Model file for the job. Use its own axes, mm. Give positions to 0.01 mm unless a question says otherwise; leave off trailing zeros. Loops run counter-clockwise (first coordinate to the right, second up) from the corner with the lowest first, then second, coordinate; pieces in that order, holes last. Notation, with made-up numbers: (-29, 0) -> (-20, 0) arc R20 cw to (-20, 23) -> close; hole circle Ø11 at (33.25, -10.5). An arc over 180 degrees is marked (long way). Use CSV: the item, a comma, the result in double quotes. Start each with the question number.
(1) Flat gauge pins, fed straight in: pin 1 (3.5 mm diameter, centred on x = -2.88, y = -6.38, fed in from -Z); pin 2 (8 mm diameter, centred on y = -72.5, z = 27.5, fed in from -X); pin 3 (13.5 mm diameter, centred on x = 21.5, y = -71, fed in from +Z). Where does each tip first touch, or does it go through?
(2) Cut at B-B on x = 21. Write the cut outline in (y, z), then the cut area to 3 significant figures.
(3) Drill centre lines: probe 1 along Z at (x, y) = (-14, -10); probe 2 along Y at (x, z) = (90.5, 5); probe 3 along Y at (x, z) = (67, -17). Where is each one in solid material? Low to high.
(4) Cut at A-A on x = -17. Write the cut outline in (y, z), then the cut area to 3 significant figures.
from build123d import *

# Parameters (mm, degrees)
SKETCH2_R           = 10
SKETCH2_R_2         = 1.275
BOSS_EXTRUDE1_DEPTH = 3
SKETCH3_R           = 1.275
BOSS_EXTRUDE2_DEPTH = 5
BOSS_EXTRUDE3_DEPTH = 5


with BuildPart() as part:
    # Sketch2 → Boss-Extrude1 (new body)
    with BuildSketch(Plane.XY):
        Circle(SKETCH2_R)
        with Locations((2.883236265, 6.378632192)):
            Circle(SKETCH2_R_2, mode=Mode.SUBTRACT)
        with Locations((6.378632192, -2.883236265)):
            Circle(SKETCH2_R_2, mode=Mode.SUBTRACT)
        with Locations((-2.883236265, -6.378632192)):
            Circle(SKETCH2_R_2, mode=Mode.SUBTRACT)
        with Locations((-6.378632192, 2.883236265)):
            Circle(SKETCH2_R_2, mode=Mode.SUBTRACT)
    extrude(amount=BOSS_EXTRUDE1_DEPTH)

    # Sketch3 → Boss-Extrude2 (add)
    with BuildSketch(Plane.XY.offset(3)):
        with BuildLine():
            Line((11.390414628, -5.148636188), (-13.323039072, -59.822626404))
            Line((-13.323039072, -59.822626404), (-36.103868329, -49.525354029))
            Line((-36.103868329, -49.525354029), (-11.390414628, 5.148636188))
            ThreePointArc((-11.390414628, 5.148636188), (5.148636188, 11.390414628), (11.390414628, -5.148636188))
        make_face()
        with Locations((2.883236265, 6.378632192)):
            Circle(SKETCH3_R, mode=Mode.SUBTRACT)
        with Locations((6.378632192, -2.883236265)):
            Circle(SKETCH3_R, mode=Mode.SUBTRACT)
        with Locations((-2.883236265, -6.378632192)):
            Circle(SKETCH3_R, mode=Mode.SUBTRACT)
        with Locations((-6.378632192, 2.883236265)):
            Circle(SKETCH3_R, mode=Mode.SUBTRACT)
    extrude(amount=-BOSS_EXTRUDE2_DEPTH)

    # Sketch4 → Boss-Extrude3 (add)
    with BuildSketch(Plane(origin=(-24.7134537, -54.673990217, 0), x_dir=(-0.91123317, 0.411890895, 0), z_dir=(-0.411890895, -0.91123317, 0))):
        with BuildLine():
            Line((-64.737964533, -30.42203086), (-34.115083994, -30.42203086))
            Line((-34.115083994, -30.42203086), (12.5, -14.551275179))
            Line((12.5, -14.551275179), (12.5, -3))
            Line((12.5, -3), (-12.5, -3))
            Line((-12.5, -3), (-42.101583528, -13.07827209))
            Line((-42.101583528, -13.07827209), (-64.737964533, -2.10203086))
            add(Edge.make_bspline(
                [(-64.737964533, -2.10203086), (-81.761805894, 22.419892021), (-132.619227666, 37.649465731), (-139.381607577, -8.76203086)],
                knots=[0, 0, 0, 0, 1, 1, 1, 1], degree=3))
            Line((-139.381607577, -8.76203086), (-139.381607577, -23.76203086))
            add(Edge.make_bspline(
                [(-64.737964533, -30.42203086), (-81.761805894, -54.943953742), (-132.619227666, -70.173527452), (-139.381607577, -23.76203086)],
                knots=[0, 0, 0, 0, 1, 1, 1, 1], degree=3))
        make_face()
    extrude(amount=-BOSS_EXTRUDE3_DEPTH)


solid = part.part
Check result:
1,pin 1,"z = -2"
1,pin 2,"x = 5.87"
1,pin 3,"z = 30.42"
2,outline,"(-75.34, 9.17) -> (-69.85, 10.26) -> (-69.85, 30.42) -> (-75.34, 30.42) -> close"
2,area,"114 mm²"
3,probe 1,"-2 to 3"
3,probe 2,"-106.75 to -101.27"
3,probe 3,"-96.13 to -90.64"
4,outline,"(-58.16, -2) -> (-7.26, -2) -> (-7.26, 3) -> (-52.67, 3) -> (-52.67, 20.92) -> (-58.16, 21.69) -> close"
4,area,"355 mm²"
